Source: CAD feature listing. Evaluate the final solid. Frame: model axes, mm. A direction names the side the tool comes from. Give positions to 0.01 mm unless a question says otherwise; leave off trailing zeros. Order: outer loops, then holes, each group sorted by start corner. A loop starts at its lowest first (then second) coordinate and runs counter-clockwise, first axis right, second up. Notation, with made-up numbers: M 78,-12.75 L 125,-12.75 A23 cw 125,0.25 Z; hole C -38,53 d9. An arc over 180 degrees is marked long. Answer in a Markdown table with one row per item. Add a question column.
(1) Section query C-C, the plane x = -18. Return loops of the section in (y, z).
(2) Section query A-A, the plane z = 5. Return loops of the section in (x, y) (3 decimals), plus the area to 3 significant figures.
(3) Mould query, pull axis Y, two halves, no side actions, for faces 6 (the face through (7.975, 53, 24)), 7 (the face through (-11, 60, 24)), 8 (the face through (-7.025, 50, 25)). Classes: pulls with the +Y half, pulls with the -Y half, needs draft (parallel to the pull), parting line crosses it, or undercut.
(4) Pin query (flat end, axial travel): P1, Ø1.5, axis at y = 53, z = 24, coming from the +X side (3 decimals); P2, Ø3.5, axis at x = -9.5, y = 48.5, coming from the +Z side; P3, Ø1, axis at x = -34.5, z = 14.5, coming from the +Y side; P4, Ø1.5, axis at x = 3, y = 49.5, coming from the +Z side. Return the tip coordinate at first contact, or that it passes through.
(5) Section query D-D, the plane z = 24.5. Return loops of the section in (x, y) (3 decimals).
(6) Section query B-B, the plane y = 53.35. Return loops of the section in (x, z) (3 decimals), plus the area to 4 significant figures.
(7) Set-up query: faces 1 (the face through (0, 36, 0)), 2 (the face through (0.37, 55.74, 23.97)), 3 (the face through (-11, 50, 14.5)), 4 (the face through (-14.025, 50, 25)), 5 (the face through (-11, 50, 34.5)). Return all of +Z, -Z, +X, -X, +Y, -Y with unobstructed straight access to the full face (end or side cutting, diameter ignored); none if empty.
(8) Material intervals for line 1 along X through (y, z) = (55, 29.5) (3 decimals); line 2 along Z through (x, y) = (-12, 45); line 3 along Y through (x, z) = (0.5, 21.5), sorted ascending.
from build123d import *

# Parameters (mm, degrees)
SKETCH1_W           = 80
SKETCH1_H           = 80
BOSS_EXTRUDE1_DEPTH = 40
SKETCH2_W           = 12.05
SKETCH2_H           = 80
CUT_EXTRUDE1_DEPTH  = 8
SKETCH3_W           = 7
SKETCH3_H           = 20
BOSS_EXTRUDE2_DEPTH = 20
SKETCH4_R           = 2.45
BOSS_EXTRUDE3_DEPTH = 15
SKETCH6_W           = 80
SKETCH6_H           = 40
CUT_EXTRUDE3_DEPTH  = 30
SKETCH7_W           = 50
SKETCH7_H           = 40
CUT_EXTRUDE4_DEPTH  = 30
SKETCH8_W           = 12.05
SKETCH8_H           = 10
BOSS_EXTRUDE4_DEPTH = 8


with BuildPart() as part:
    # Sketch1 → Boss-Extrude1 (new body)
    with BuildSketch(Plane(origin=(0, 0, 0), x_dir=(1, 0, 0), z_dir=(0, 1, 0))):
        Rectangle(SKETCH1_W, SKETCH1_H)
    extrude(amount=BOSS_EXTRUDE1_DEPTH)

    # Sketch2 → Cut-Extrude1 (cut)
    with BuildSketch(Plane(origin=(0, 40, 0), x_dir=(1, 0, 0), z_dir=(0, 1, 0))):
        Rectangle(SKETCH2_W, SKETCH2_H)
    extrude(amount=-CUT_EXTRUDE1_DEPTH, mode=Mode.SUBTRACT)

    # Sketch3 → Boss-Extrude2 (add)
    with BuildSketch(Plane(origin=(0, 40, 0), x_dir=(1, 0, 0), z_dir=(0, 1, 0))):
        with Locations((-10.525, -24.5)):
            Rectangle(SKETCH3_W, SKETCH3_H)
    extrude(amount=BOSS_EXTRUDE2_DEPTH)

    # Sketch4 → Boss-Extrude3 (add)
    with BuildSketch(Plane(origin=(-7.025, 0, 0), x_dir=(0, 0, -1), z_dir=(1, 0, 0))):
        with Locations(Location((-24.5, 53.35, 0), (0, 0, 180))):
            Circle(SKETCH4_R)
    extrude(amount=BOSS_EXTRUDE3_DEPTH)

    # Sketch6 → Cut-Extrude3 (cut)
    with BuildSketch(Plane(origin=(0, 0, -40), x_dir=(-1, 0, 0), z_dir=(0, 0, -1))):
        with Locations((0, 20)):
            Rectangle(SKETCH6_W, SKETCH6_H)
    extrude(amount=-CUT_EXTRUDE3_DEPTH, mode=Mode.SUBTRACT)

    # Sketch7 → Cut-Extrude4 (cut)
    with BuildSketch(Plane(origin=(40, 0, 0), x_dir=(0, 0, -1), z_dir=(1, 0, 0))):
        with Locations((-15, 20)):
            Rectangle(SKETCH7_W, SKETCH7_H)
    extrude(amount=-CUT_EXTRUDE4_DEPTH, mode=Mode.SUBTRACT)

    # Sketch8 → Boss-Extrude4 (add)
    with BuildSketch(Plane(origin=(0, 32, 0), x_dir=(1, 0, 0), z_dir=(0, 1, 0))):
        with Locations((0, 5)):
            Rectangle(SKETCH8_W, SKETCH8_H)
    extrude(amount=BOSS_EXTRUDE4_DEPTH)


solid = part.part
Values follow:
| question | item | result |
|---|---|---|
| 1 | outline | M 0,-10 L 40,-10 L 40,40 L 0,40 Z |
| 2 | outline | M -40,0 L 10,0 L 10,40 L 6.025,40 L 6.025,32 L -6.025,32 L -6.025,40 L -40,40 Z |
| 2 | area | 1,900 mm² |
| 3 | face 6 | needs draft |
| 3 | face 7 | pulls with the +Y half |
| 3 | face 8 | undercut |
| 4 | P1 | stops at x = 7.975 |
| 4 | P2 | stops at z = 34.5 |
| 4 | P3 | stops at y = 40 |
| 4 | P4 | passes through |
| 5 | outline | M -40,0 L 10,0 L 10,40 L 6.025,40 L 6.025,32 L -6.025,32 L -6.025,40 L -7.025,40 L -7.025,50.9 L 7.975,50.9 L 7.975,55.8 L -7.025,55.8 L -7.025,60 L -14.025,60 L -14.025,40 L -40,40 Z |
| 6 | outline | M -14.025,14.5 L -7.025,14.5 L -7.025,22.05 L 7.975,22.05 L 7.975,26.95 L -7.025,26.95 L -7.025,34.5 L -14.025,34.5 Z |
| 6 | area | 213.5 mm² |
| 7 | face 1 | +Z, +Y |
| 7 | face 2 | +X |
| 7 | face 3 | -Z, +X, -X, +Y |
| 7 | face 4 | +Z, -Z, -X, +Y |
| 7 | face 5 | +Z, +X, -X, +Y |
| 8 | line 1 | x = -14.025 to -7.025 |
| 8 | line 2 | z = 14.5 to 34.5 |
| 8 | line 3 | y = 0 to 32 |
